```python
from build123d import *

# Parameters (mm, degrees)
SKETCH_1_R          = 2
EXTRUDE_1_DEPTH     = 5
SKETCH_2_R          = 7.5
CUT_EXTRUDE_1_DEPTH = 10
SKETCH_3_W          = 8
SKETCH_3_H          = 40
CUT_EXTRUDE_2_DEPTH = 71.185468581
SKETCH_6_R          = 1.5
CUT_EXTRUDE_3_DEPTH = 71.185468581
SKETCH_7_R          = 4.5
SKETCH_7_R_2        = 1.5
CUT_EXTRUDE_4_DEPTH = 2
SKETCH_8_W          = 3
SKETCH_8_H          = 45
CUT_EXTRUDE_5_DEPTH = 71.185468581
SKETCH_9_R          = 1.5
CUT_EXTRUDE_6_DEPTH = 10
SKETCH_10_R         = 1.5
CUT_EXTRUDE_7_DEPTH = 10


with BuildPart() as part:
    # 草图1 → 凸台-拉伸1 (new body)
    with BuildSketch(Plane.XY):
        Polygon((-25, 50), (25, 50), (25, 32.424322584), (25, 0), (49, 0), (49, -50), (25, -50), (-25, -50), (-49, -50), (-49, 0), (-25, 0), (-25, 32.424322584), align=None)
        with Locations((-15, 44)):
            Circle(SKETCH_1_R, mode=Mode.SUBTRACT)
        with Locations(Location((15, 44, 0), (0, 0, 180))):
            Circle(SKETCH_1_R, mode=Mode.SUBTRACT)
    extrude(amount=EXTRUDE_1_DEPTH)

    # 草图2 → 切除-拉伸1 (cut)
    with BuildSketch(Plane.XY.offset(5)):
        with Locations((0, 44)):
            Circle(SKETCH_2_R)
    extrude(amount=-CUT_EXTRUDE_1_DEPTH, mode=Mode.SUBTRACT)

    # 草图3 → 切除-拉伸2 (cut, through all)
    with BuildSketch(Plane(origin=(0, 0, 0), x_dir=(-1, 0, 0), z_dir=(0, 0, -1))):
        with Locations((0, -30)):
            Rectangle(SKETCH_3_W, SKETCH_3_H)
    extrude(amount=-CUT_EXTRUDE_2_DEPTH, mode=Mode.SUBTRACT)

    # 草图6 → 切除-拉伸3 (cut, through all)
    with BuildSketch(Plane(origin=(0, 0, 0), x_dir=(-1, 0, 0), z_dir=(0, 0, -1))):
        with Locations(Location((-32.235018023, -44, 0), (0, 0, 180))):
            Circle(SKETCH_6_R)
        with Locations(Location((-32.235018023, -20, 0), (0, 0, 180))):
            Circle(SKETCH_6_R)
        with Locations((32.235018023, -44)):
            Circle(SKETCH_6_R)
        with Locations((32.235018023, -20)):
            Circle(SKETCH_6_R)
    extrude(amount=-CUT_EXTRUDE_3_DEPTH, mode=Mode.SUBTRACT)

    # 草图7 → 切除-拉伸4 (cut)
    # profile 1 of 4: a face of its own
    with BuildSketch(Plane(origin=(0, 0, 0), x_dir=(-1, 0, 0), z_dir=(0, 0, -1))):
        with Locations((-32.235018023, -44)):
            Circle(SKETCH_7_R)
        with Locations((-32.235018023, -44)):
            Circle(SKETCH_7_R_2, mode=Mode.SUBTRACT)
    # profile 2 of 4: a face of its own
    with BuildSketch(Plane(origin=(0, 0, 0), x_dir=(-1, 0, 0), z_dir=(0, 0, -1))):
        with Locations((-32.235018023, -20)):
            Circle(SKETCH_7_R)
        with Locations((-32.235018023, -20)):
            Circle(SKETCH_7_R_2, mode=Mode.SUBTRACT)
    # profile 3 of 4: a face of its own
    with BuildSketch(Plane(origin=(0, 0, 0), x_dir=(-1, 0, 0), z_dir=(0, 0, -1))):
        with Locations((32.235018023, -20)):
            Circle(SKETCH_7_R)
        with Locations((32.235018023, -20)):
            Circle(SKETCH_7_R_2, mode=Mode.SUBTRACT)
    # profile 4 of 4: a face of its own
    with BuildSketch(Plane(origin=(0, 0, 0), x_dir=(-1, 0, 0), z_dir=(0, 0, -1))):
        with Locations((32.235018023, -44)):
            Circle(SKETCH_7_R)
        with Locations((32.235018023, -44)):
            Circle(SKETCH_7_R_2, mode=Mode.SUBTRACT)
    extrude(amount=-CUT_EXTRUDE_4_DEPTH, mode=Mode.SUBTRACT)

    # 草图8 → 切除-拉伸5 (cut, through all)
    with BuildSketch(Plane(origin=(0, 0, 0), x_dir=(-1, 0, 0), z_dir=(0, 0, -1))):
        with Locations((-15.035926406, -17.789740129)):
            Rectangle(SKETCH_8_W, SKETCH_8_H)
    extrude(amount=-CUT_EXTRUDE_5_DEPTH, mode=Mode.SUBTRACT)

    # 草图9 → 切除-拉伸6 (cut)
    with BuildSketch(Plane(origin=(0, 0, 0), x_dir=(-1, 0, 0), z_dir=(0, 0, -1))):
        with Locations((-4.5, 10.25)):
            Circle(SKETCH_9_R)
        with Locations(Location((4.5, 10.25, 0), (0, 0, 180))):
            Circle(SKETCH_9_R)
    extrude(amount=-CUT_EXTRUDE_6_DEPTH, mode=Mode.SUBTRACT)

    # 草图10 → 切除-拉伸7 (cut)
    with BuildSketch(Plane(origin=(0, 0, 0), x_dir=(-1, 0, 0), z_dir=(0, 0, -1))):
        with Locations((9.5, -22.5)):
            Circle(SKETCH_10_R)
        with Locations((19.5, -22.5)):
            Circle(SKETCH_10_R)
        with Locations((19.5, -37.5)):
            Circle(SKETCH_10_R)
        with Locations((9.5, -37.5)):
            Circle(SKETCH_10_R)
    extrude(amount=-CUT_EXTRUDE_7_DEPTH, mode=Mode.SUBTRACT)


solid = part.part
```
Design review of the part built by this model. Coordinates are the model's own, in mm. A direction names the side the tool comes from. Give positions to 0.01 mm unless a question says otherwise; leave off trailing zeros. Order: outer loops, then holes, each group sorted by start corner. A loop starts at its lowest first (then second) coordinate and runs counter-clockwise, first axis right, second up. Notation, with made-up numbers: (62.25, 55) -> (120.25, 55) arc R18 ccw to (120.25, 80) -> close; hole circle Ø2 at (-29, 17.5). An arc over 180 degrees is marked (long way). Write each question's results on one line, items separated by ' | '. Start each with the question number.
Q1. Machinability: for faces 1 (the flat face through (15, 4.71, 2)), 2 (the flat face through (30, -20, 2)), 3 (the flat face through (49, -25, 2)), which of the approach directions +Z, -Z, +X, -X, +Y, -Y give a long, thin tool a straight path to every point of the face, cutting with its end or side? Answer none if there is none.
Q2. Add section A-A on x = -9.5. Give the boundary of the cut face in (y, z), and give its area (3 significant figures).
Q3. Add section D-D on z = 3.35. State how many separate pieces and enclosed holes the cut face has, and give its area (3 significant figures).
Q4. Mouldability with a two-part tool opening along Y and no side actions: class faces 4 (the flat face through (-27, -50, 2)), 5 (the flat face through (25, 25, 2)), 6 (the flat face through (37, 0, 2)), 7 (the cylindrical face through (-9.175, -38.964, 2.465)) as +Y half, -Y half, draft (parallel to the pull), parting line (faces both ways), or undercut.
Q5. Add section B-B on y = -37.5. Give the boundary of the cut face in (x, z).
Q6. For pin 1 (3.5 mm diameter, centred on x = 15, y = 44, fed in from +Z); pin 2 (5 mm diameter, centred on x = 32.24, y = -44, fed in from -Z), all flat-tipped, find the tip position at first contact; note any pin that passes through.
Q7. Add section C-C on y = -11.5. Give the boundary of the cut face in (x, z), and give its area (3 significant figures).
Q8. Wall thickness on L1, parallel to Y at x = -9.5, z = 3.85; L2, parallel to X at y = -30, z = 4.8; L3, parallel to Y at x = 14, z = 1.9: over which ranges is each line inside the solid? List them lowest first. Write a range as from..to.
Found:
1) face 1: +Z, -Z | face 2: -Z | face 3: +Z, -Z, +X, +Y, -Y
2) outline: (-50, 0) -> (-39, 0) -> (-39, 5) -> (-50, 5) -> close; (-36, 0) -> (-24, 0) -> (-24, 5) -> (-36, 5) -> close; (-21, 0) -> (50, 0) -> (50, 5) -> (-21, 5) -> close | area: 470 mm2
3) separate pieces: 1 | enclosed holes: 13 | area: 6,680 mm2
4) face 4: -Y half | face 5: draft | face 6: +Y half | face 7: undercut
5) outline: (-49, 0) -> (-21, 0) -> (-21, 5) -> (-49, 5) -> close; (-18, 0) -> (-11, 0) -> (-11, 5) -> (-18, 5) -> close; (-8, 0) -> (-4, 0) -> (-4, 5) -> (-8, 5) -> close; (4, 0) -> (13.54, 0) -> (13.54, 5) -> (4, 5) -> close; (16.54, 0) -> (49, 0) -> (49, 5) -> (16.54, 5) -> close
6) pin 1: passes through | pin 2: stops at z = 2
7) outline: (-49, 0) -> (-4, 0) -> (-4, 5) -> (-49, 5) -> close; (4, 0) -> (13.54, 0) -> (13.54, 5) -> (4, 5) -> close; (16.54, 0) -> (49, 0) -> (49, 5) -> (16.54, 5) -> close | area: 435 mm2
8) L1: y = -50..-39, -36..-24, -21..50 | L2: x = -49..-4, 4..13.54, 16.54..49 | L3: y = -50..-40.29, 4.71..42.27, 45.73..50
